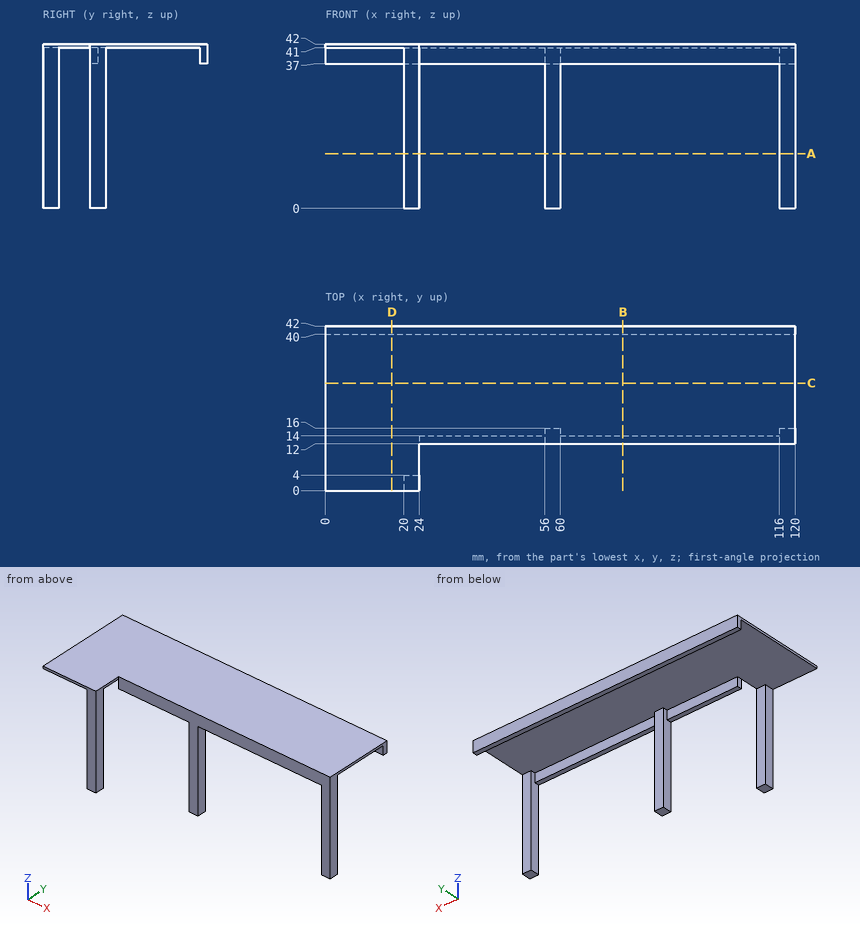
Source: three-view drawing plus pictorial views. Frame: mm from the lowest corner of the part. Give positions to 0.01 mm unless a question says otherwise; leave off trailing zeros. Loops run counter-clockwise (first coordinate to the right, second up) from the corner with the lowest first, then second, coordinate; pieces in that order, holes last. Notation, with made-up numbers: (37.5, 87) -> (50.5, 87) arc R17 cw to (50.5, 99) -> close; hole circle Ø5 at (30, 76). An arc over 180 degrees is marked (long way). Put each result on its own line as item: value. Start each with the question number.
1) Cut plane D-D (x = 17). Return loops of the section in (y, z), then the cut area to 3 significant figures.
2) Cut plane C-C (y = 27.5). Return loops of the section in (x, z), then the cut area to 3 significant figures.
3) Cut plane B-B (x = 76). Return loops of the section in (y, z).
4) Contact query for flat-ended pins moving along their axis: P1, Ø0.6, axis at x = 95, y = 13.5, coming from the -Z side; P2, Ø2, axis at x = 119, z = 20, coming from the +Y side; P3, Ø9.5, axis at y = 4.5, z = 22.5, coming from the +X side. Output: stop coordinate, or through.
5) Cut plane A-A (z = 14). Return loops of the section in (x, y), then the cut area to 3 significant figures.
6) Material intervals for probe 1 along X at (y, z) = (15, 19); probe 2 along Y at (x, z) = (63, 39); probe 3 along Z at (x, y) = (5, 26.5), sorted ascending.
Results are:
1. outline: (0, 41) -> (40, 41) -> (40, 37) -> (42, 37) -> (42, 42) -> (0, 42) -> close
1. area: 50.0 mm2
2. outline: (0, 41) -> (120, 41) -> (120, 42) -> (0, 42) -> close
2. area: 120 mm2
3. outline: (12, 37) -> (14, 37) -> (14, 41) -> (40, 41) -> (40, 37) -> (42, 37) -> (42, 42) -> (12, 42) -> close
4. P1: stops at z = 37
4. P2: stops at y = 16
4. P3: stops at x = 24
5. outline: (20, 0) -> (24, 0) -> (24, 4) -> (20, 4) -> close; (56, 12) -> (60, 12) -> (60, 16) -> (56, 16) -> close; (116, 12) -> (120, 12) -> (120, 16) -> (116, 16) -> close
5. area: 48.0 mm2
6. probe 1: x = 56 to 60, 116 to 120
6. probe 2: y = 12 to 14, 40 to 42
6. probe 3: z = 41 to 42
